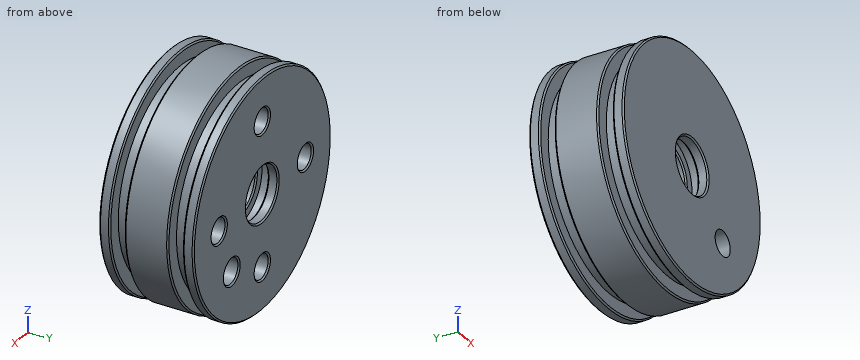
Autodesk Inventor part; units mm, degrees
ref_plane "YZ Plane" through (0, 0, 0) normal (1, 0, 0) x (0, 1, 0)
ref_plane "XZ Plane" through (0, 0, 0) normal (0, 1, 0) x (-1, 0, 0)
ref_plane "XY Plane" through (0, 0, 0) normal (0, 0, 1) x (1, 0, 0)
sketch "Sketch1" plane through (0, 0, 0) normal (0, 0, 1) x (1, 0, 0)
  line L0 (50.8, 0) -> (50.8, 39.0312) construction
  line L1 (0, 0) -> (50.6412, 0)
  line L2 (44.45, 0) -> (44.45, 51.6727)
  line L3 (0, 0) -> (0, 50.5742)
  line L4 (50.6412, 0) -> (50.6412, 45.6895)
  line L5 (50.6413, 4.7625) -> (44.45, 4.7625)
  line L6 (44.45, 11.1125) -> (50.6412, 11.1125)
  line L7 (50.6412, 30.1625) -> (44.45, 30.1625)
  line L8 (44.45, 36.5125) -> (50.6412, 36.5125)
  line L9 (50.6412, 41.275) -> (0, 41.275)
  line L10 (11.8237, 0) -> (11.8237, 53.9909)
  line L11 (15.875, 0) -> (15.875, 48.05)
  line L12 (11.8237, 4.7625) -> (15.875, 4.7625)
  line L13 (15.875, 9.5377) -> (11.8237, 9.5377)
  line L14 (15.875, 31.7373) -> (11.8237, 31.7373)
  line L15 (11.8237, 36.5125) -> (15.875, 36.5125)
  point P0 (47.5456, 36.5125)
  point P1 (44.45, 30.1625)
  point P2 (11.8237, 41.275)
  dimension "d1" = 50.6412
  dimension "d2" = 44.45
  dimension "d3" = 6.35
  dimension "d4" = 6.35
  dimension "d5" = 4.7625
  dimension "d6" = 19.05
  dimension "d7" = 4.7625
  dimension "d12" = 41.275
  dimension "d20" = 11.8237
  dimension "d22" = 15.875
  dimension "d23" = 4.7752
  dimension "d24" = 4.7752
revolve "Revolution1" add sketch "Sketch1" angle 360 about axis through (0, 0, 0) along (0, 1, 0) contours L10 L12 L11 L1 | L11 L9 L2 L1 | L9 L11 L15 L10 | L2 L5 L4 L1 | L10 L14 L11 L13 | L9 L4 L8 L2 | L2 L7 L4 L6
chamfer "Chamfer1" distance 0.635 angle 45 12 edges at (-50.6412, 0, 0) (-50.6413, 4.7625, 0) (-50.6412, 11.1125, 0) (-50.6412, 30.1625, 0) (-50.6412, 36.5125, 0) (-50.6412, 41.275, 0) (-11.8237, 41.275, 0) (-11.8237, 36.5125, 0) (-11.8237, 31.7373, 0) (-11.8237, 9.5377, 0) (-11.8237, 4.7625, 0) (-11.8237, 0, 0)
sketch "Sketch3" plane through (0, 41.275, 0) normal (0, 1, 0) x (1, 0, 0)
  circle A0 centre (0, 31.75) radius 5.3578
  circle A1 centre (-31.75, 0) radius 5.3578
  circle A2 centre (0, -31.75) radius 5.3578
  circle A3 centre (31.75, 0) radius 5.3578
  circle A4 centre (0, 0) radius 31.75 construction
  line L0 (0, 0) -> (22.4506, 22.4506) construction
  line L1 (0, 0) -> (31.75, 0) construction
  circle A5 centre (22.4506, 22.4506) radius 5.5563
  dimension "d27" = 360
  dimension "d29" = 10.7156
  dimension "d30" = 31.75
  dimension "d31" = 45
  dimension "d32" = 11.1125
extrude "Extrusion3" cut sketch "Sketch3" against normal up to surface (30.1625 mm away) contours A0 | A1 | A2 | A3
extrude "Extrusion4" cut sketch "Sketch3" against normal blind 352.425 contours A5
chamfer "Chamfer2" distance 0.635 angle 45 5 edges at (-37.1078, 41.275, 0) (-5.3578, 41.275, -31.75) (16.8944, 41.275, -22.4506) (26.3922, 41.275, 0) (-5.3578, 41.275, 31.75)
properties part number "2 Piston"
Can you work these out from the model? Positions are in its coordinate system, mm. Give positions to 0.01 mm unless a question says otherwise; leave off trailing zeros. Loops run counter-clockwise (first coordinate to the right, second up) from the corner with the lowest first, then second, coordinate; pieces in that order, holes last. Notation, with made-up numbers: M -19,-5 L 30,-5 A33 ccw 30,31 Z; hole C 28.25,-6.5 d8. An arc over 180 degrees is marked long. Use one line per item in the form item = value. Start each with the question number.
(1) I want a section at B-B, the plane x = -14.5. State how many separate pieces and enclosed holes the cut face has, and give its area (3 significant figures).
(2) Please list where these lines run through material, in increasing order: line 1 (X direction, y = 16, z = 0); line 2 (Y direction, x = -23, z = 41) (1 decimal); line 3 (X direction, y = 34.4, z = 0) (3 decimals).
(3) I want a section at A-A, the plane y = 18.5. Write out the boundary of the cut face in (x, z).
(4) I'm going to push flat-ended pins straight in: P1, Ø10, axis at x = 34.5, y = 34.5, coming from the +Z side; P2, Ø12, axis at y = 16, z = -35.5, coming from the +X side; P3, Ø6, axis at x = -10.5, z = -40, coming from the -Y side; P4, Ø10, axis at x = -22.5, y = 17.5, coming from the -Z side. Where does each tip first touch, or does it pass through?
Worked out:
q1.separate_pieces = 1
q1.enclosed_holes = 2
q1.area = 3,710 mm²
q2.line_1 = -50.64 to -37.11, -26.39 to -11.82, 11.82 to 26.39, 37.11 to 50.64
q2.line_2 = 0 to 4.8, 11.1 to 30.2, 36.5 to 41.3
q2.line_3 = -44.45 to -37.108, -26.392 to -15.875, 15.875 to 26.392, 37.108 to 44.45
q3.outline = C 0,0 d101.28; hole C -31.75,0 d10.72; hole C 0,0 d23.65; hole C 0,-31.75 d10.72; hole C 0,31.75 d10.72; hole C 22.45,-22.45 d11.11; hole C 31.75,0 d10.72
q4.P1 = 40.61
q4.P2 = 41.16
q4.P3 = 0
q4.P4 = -47.52
